```python
from build123d import *

# Parameters (mm, degrees)
CUT_EXTRUDE1_DEPTH = 4
FILLET1_R          = 0.5


with BuildPart() as part:
    # Sketch1 → Revolve1 (revolve)
    with BuildSketch(Plane.XY, mode=Mode.PRIVATE) as revolve1_sk:
        Polygon((0, 13.05), (0, -13.05), (4, -13.05), (4, 6.95), (1, 6.95), (1, 8.95), (2, 8.95), (2, 12.95), (1, 12.95), (1, 13.05), align=None)
    revolve(revolve1_sk.sketch.rotate(Axis((0, 13.05, 0), (0, -1, 0)), 180), axis=Axis((0, 13.05, 0), (0, -1, 0)))

    # Sketch2 → Cut-Extrude1 (cut)
    with BuildSketch(Plane(origin=(0, 12.95, 0), x_dir=(1, 0, 0), z_dir=(0, 1, 0))):
        with BuildLine():
            ThreePointArc((0.5, 1.936491673), (0, 2), (-0.5, 1.936491673))
            ThreePointArc((-0.5, 1.936491673), (-0.264591418, 1.626479536), (-0.093693162, 1.276738901))
            ThreePointArc((-0.093693162, 1.276738901), (0, 1.211690173), (0.093693162, 1.276738901))
            ThreePointArc((0.093693162, 1.276738901), (0.264591418, 1.626479536), (0.5, 1.936491673))
        make_face()
        with BuildLine():
            ThreePointArc((1.467573208, 1.358760053), (1.101929691, 1.225232735), (0.769076867, 1.023406763))
            ThreePointArc((0.769076867, 1.023406763), (0.655089165, 1.019338638), (0.61143746, 1.124715459))
            ThreePointArc((0.61143746, 1.124715459), (0.65675276, 1.511330576), (0.626319675, 1.89940087))
            ThreePointArc((0.626319675, 1.89940087), (1.081281635, 1.682507066), (1.467573208, 1.358760053))
        make_face()
        with BuildLine():
            ThreePointArc((1.969202291, 0.349631716), (1.589413073, 0.434983198), (1.2002841, 0.445150209))
            ThreePointArc((1.2002841, 0.445150209), (1.102192149, 0.503354289), (1.122441008, 0.615602805))
            ThreePointArc((1.122441008, 0.615602805), (1.369582578, 0.916344837), (1.553787278, 1.259263711))
            ThreePointArc((1.553787278, 1.259263711), (1.819263991, 0.830830026), (1.969202291, 0.349631716))
        make_face()
        with BuildLine():
            ThreePointArc((1.845623561, -0.77050222), (1.572269034, -0.493370431), (1.250409613, -0.274438391))
            ThreePointArc((1.250409613, -0.274438391), (1.199356914, -0.172441491), (1.277077467, -0.088959389))
            ThreePointArc((1.277077467, -0.088959389), (1.647579604, 0.030426087), (1.987938399, 0.219319222))
            ThreePointArc((1.987938399, 0.219319222), (1.979642884, -0.284629677), (1.845623561, -0.77050222))
        make_face()
        with BuildLine():
            ThreePointArc((1.136072391, -1.646007146), (1.055940687, -1.265082434), (0.903538908, -0.906894741))
            ThreePointArc((0.903538908, -0.906894741), (0.915734332, -0.793488316), (1.026250854, -0.765277606))
            ThreePointArc((1.026250854, -0.765277606), (1.402481747, -0.865152731), (1.790933125, -0.890257571))
            ThreePointArc((1.790933125, -0.890257571), (1.511499149, -1.309721468), (1.136072391, -1.646007146))
        make_face()
        with BuildLine():
            ThreePointArc((0.065826264, -1.998916432), (0.204358632, -1.635139703), (0.269800984, -1.251418419))
            ThreePointArc((0.269800984, -1.251418419), (0.34137257, -1.162608207), (0.449596846, -1.198625591))
            ThreePointArc((0.449596846, -1.198625591), (0.712105845, -1.48605167), (1.025319237, -1.717183875))
            ThreePointArc((1.025319237, -1.717183875), (0.563465114, -1.918985947), (0.065826264, -1.998916432))
        make_face()
        with BuildLine():
            ThreePointArc((-1.025319237, -1.717183875), (-0.712105845, -1.48605167), (-0.449596846, -1.198625591))
            ThreePointArc((-0.449596846, -1.198625591), (-0.34137257, -1.162608207), (-0.269800984, -1.251418419))
            ThreePointArc((-0.269800984, -1.251418419), (-0.204358632, -1.635139703), (-0.065826264, -1.998916432))
            ThreePointArc((-0.065826264, -1.998916432), (-0.563465114, -1.918985947), (-1.025319237, -1.717183875))
        make_face()
        with BuildLine():
            ThreePointArc((-1.790933125, -0.890257571), (-1.402481747, -0.865152731), (-1.026250854, -0.765277606))
            ThreePointArc((-1.026250854, -0.765277606), (-0.915734332, -0.793488316), (-0.903538908, -0.906894741))
            ThreePointArc((-0.903538908, -0.906894741), (-1.055940687, -1.265082434), (-1.136072391, -1.646007146))
            ThreePointArc((-1.136072391, -1.646007146), (-1.511499149, -1.309721468), (-1.790933125, -0.890257571))
        make_face()
        with BuildLine():
            ThreePointArc((-1.987938399, 0.219319222), (-1.647579604, 0.030426087), (-1.277077467, -0.088959389))
            ThreePointArc((-1.277077467, -0.088959389), (-1.199356914, -0.172441491), (-1.250409613, -0.274438391))
            ThreePointArc((-1.250409613, -0.274438391), (-1.572269034, -0.493370431), (-1.845623561, -0.77050222))
            ThreePointArc((-1.845623561, -0.77050222), (-1.979642884, -0.284629677), (-1.987938399, 0.219319222))
        make_face()
        with BuildLine():
            ThreePointArc((-1.553787278, 1.259263711), (-1.369582578, 0.916344837), (-1.122441008, 0.615602805))
            ThreePointArc((-1.122441008, 0.615602805), (-1.102192149, 0.503354289), (-1.2002841, 0.445150209))
            ThreePointArc((-1.2002841, 0.445150209), (-1.589413073, 0.434983198), (-1.969202291, 0.349631716))
            ThreePointArc((-1.969202291, 0.349631716), (-1.819263991, 0.830830026), (-1.553787278, 1.259263711))
        make_face()
        with BuildLine():
            ThreePointArc((-0.626319675, 1.89940087), (-0.65675276, 1.511330576), (-0.61143746, 1.124715459))
            ThreePointArc((-0.61143746, 1.124715459), (-0.655089165, 1.019338638), (-0.769076867, 1.023406763))
            ThreePointArc((-0.769076867, 1.023406763), (-1.101929691, 1.225232735), (-1.467573208, 1.358760053))
            ThreePointArc((-1.467573208, 1.358760053), (-1.081281635, 1.682507066), (-0.626319675, 1.89940087))
        make_face()
    extrude(amount=-CUT_EXTRUDE1_DEPTH, mode=Mode.SUBTRACT)

    # Fillet1
    fillet1_edges = [part.edges().sort_by_distance(p)[0] for p in [
        (4, -13.05, 0),
        (4, 6.95, 0),
    ]]
    fillet(fillet1_edges, radius=FILLET1_R)


solid = part.part
```
Source: CAD feature listing. Evaluate the final solid. Frame: model axes, mm. A direction names the side the tool comes from. Give positions to 0.01 mm unless a question says otherwise; leave off trailing zeros. Loops run counter-clockwise (first coordinate to the right, second up) from the corner with the lowest first, then second, coordinate; pieces in that order, holes last. Notation, with made-up numbers: (47.5, 21.25) - (89.5, 21.25) arc R13 cw to (89.5, 40.25) - close; hole circle Ø2 at (31, 10). An arc over 180 degrees is marked (long way). Use CSV: the item, a comma, the result in double quotes. Start each with the question number.
1. Pin query (flat end, axial travel): pin 1 (3 mm diameter, centred on y = -4, z = -0.5, fed in from +X); pin 2 (3 mm diameter, centred on x = 2.5, z = -3, fed in from +Y); pin 3 (4 mm diameter, centred on x = -2.5, y = 7.5, fed in from -Z); pin 4 (1.5 mm diameter, centred on x = 0, z = 2, fed in from +Y). Return the tip coordinate at first contact, or that it passes through.
2. Reachability of faces 1 (the flat face through (-1, 6.95, 1)), 2 (the flat face through (0, 13.05, 0)) from +Z, -Z, +X, -X, +Y, -Y: full face, straight path, thin tool, end or side. Return the list, or none.
3. Draft query along Y for faces 3 (the cylindrical face through (0, 8, 1)), 4 (the flat face through (0, -13.05, 0)), 5 (the cylindrical face through (0.867, -2.917, 3.905)). Return one class per face: +Y half, -Y half, draft (parallel to the pull), parting line (faces both ways), or undercut.
4. Section A-A (y = 7.25). Output: boundary loops of the cut face in (x, z).
5. Section B-B (y = -7). Output: boundary loops of the cut face in (x, z).
6. Ray query, L1, parallel to Y at x = 2.5, z = 0.5; L2, parallel to Z at x = -1.5, y = -9.75. Return the intervals inside material, ascending.
Response:
1,pin 1,"x = 4"
1,pin 2,"y = 6.95"
1,pin 3,"z = -3.92"
1,pin 4,"y = 12.95"
2,face 1,"none"
2,face 2,"+Z, -Z, +X, -X, +Y"
3,face 3,"undercut"
3,face 4,"-Y half"
3,face 5,"draft"
4,outline,"circle Ø2 at (0, 0)"
5,outline,"circle Ø8 at (0, 0)"
6,L1,"-13.05 to 6.95"
6,L2,"-3.71 to 3.71"
